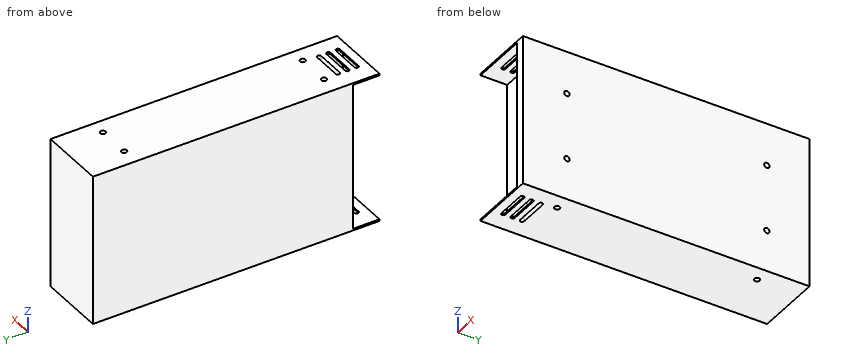
```python
from build123d import *

# Parameters (mm, degrees)
ESBO_O1_W                = 50
ESBO_O1_H                = 215
RESSALTO_EXTRUS_O1_DEPTH = 113
CORTE_EXTRUS_O1_DEPTH    = 113
ESBO_O3_W                = 110.4
ESBO_O3_H                = 20
CORTE_EXTRUS_O2_DEPTH    = 43
ESBO_O4_R                = 2
CORTE_EXTRUS_O3_DEPTH    = 113
ESBO_O5_R                = 2
CORTE_EXTRUS_O4_DEPTH    = 10
ESBO_O6_R                = 2
CORTE_EXTRUS_O5_DEPTH    = 10


with BuildPart() as part:
    # Esboço1 → Ressalto-extrusão1 (new body)
    with BuildSketch(Plane.XY):
        Rectangle(ESBO_O1_W, ESBO_O1_H)
    extrude(amount=RESSALTO_EXTRUS_O1_DEPTH)

    # Esboço2 → Corte-extrusão1 (cut)
    with BuildSketch(Plane(origin=(0, 0, 0), x_dir=(-1, 0, 0), z_dir=(0, 0, -1))):
        with BuildLine():
            Line((-11.5, -98), (10.5, -98))
            ThreePointArc((10.5, -98), (12, -99.5), (10.5, -101))
            Line((10.5, -101), (-11.5, -101))
            ThreePointArc((-11.5, -101), (-13, -99.5), (-11.5, -98))
        make_face()
        with BuildLine():
            Line((-11.5, -91), (10.5, -91))
            ThreePointArc((10.5, -91), (12, -92.5), (10.5, -94))
            Line((10.5, -94), (-11.5, -94))
            ThreePointArc((-11.5, -94), (-13, -92.5), (-11.5, -91))
        make_face()
        with BuildLine():
            Line((-11.5, -84), (10.5, -84))
            ThreePointArc((10.5, -84), (12, -85.5), (10.5, -87))
            Line((10.5, -87), (-11.5, -87))
            ThreePointArc((-11.5, -87), (-13, -85.5), (-11.5, -84))
        make_face()
    extrude(amount=-CORTE_EXTRUS_O1_DEPTH, mode=Mode.SUBTRACT)

    # Esboço3 → Corte-extrusão2 (cut)
    with BuildSketch(Plane.ZY.offset(25)):
        with Locations((56.5, -97.5)):
            Rectangle(ESBO_O3_W, ESBO_O3_H)
    extrude(amount=-CORTE_EXTRUS_O2_DEPTH, mode=Mode.SUBTRACT)

    # Esboço4 → Corte-extrusão3 (cut)
    with BuildSketch(Plane.XY.offset(113)):
        with Locations((13.5, -74.5)):
            Circle(ESBO_O4_R)
        with Locations((13.5, 75.5)):
            Circle(ESBO_O4_R)
    extrude(amount=-CORTE_EXTRUS_O3_DEPTH, mode=Mode.SUBTRACT)

    # Esboço5 → Corte-extrusão4 (cut)
    with BuildSketch(Plane.XY.offset(113)):
        with Locations((-11.5, 75.5)):
            Circle(ESBO_O5_R)
        with Locations((-11.5, -74.5)):
            Circle(ESBO_O5_R)
    extrude(amount=-CORTE_EXTRUS_O4_DEPTH, mode=Mode.SUBTRACT)

    # Esboço6 → Corte-extrusão5 (cut)
    with BuildSketch(Plane(origin=(25, 0, 0), x_dir=(0, 0, -1), z_dir=(1, 0, 0))):
        with Locations((-31, -74.5)):
            Circle(ESBO_O6_R)
        with Locations((-81, -74.5)):
            Circle(ESBO_O6_R)
        with Locations((-31, 75.5)):
            Circle(ESBO_O6_R)
        with Locations((-81, 75.5)):
            Circle(ESBO_O6_R)
    extrude(amount=-CORTE_EXTRUS_O5_DEPTH, mode=Mode.SUBTRACT)


solid = part.part
```
Source: CAD feature listing. Evaluate the final solid. Frame: model axes, mm. Coordinates: 2 decimals unless noted, no trailing zeros. Loops run counter-clockwise (first coordinate to the right, second up) from the corner with the lowest first, then second, coordinate; pieces in that order, holes last. Notation, with made-up numbers: (33.25, 49.5) - (63.25, 49.5) arc R9 cw to (63.25, 65.5) - close; hole circle Ø5 at (71, 10). An arc over 180 degrees is marked (long way). Answer as CSV lines item,"result".
1. Contact query for flat-ended pins moving along their axis: pin 1 (10 mm diameter, centred on x = -3.5, y = -99, fed in from -Z); pin 2 (24 mm diameter, centred on x = -3, z = 52.5, fed in from -Y); pin 3 (0.5 mm diameter, centred on y = 74, z = 31, fed in from +X); pin 4 (16 mm diameter, centred on y = -99, z = 38, fed in from -X). Output: stop coordinate, or through.
Established:
pin 1,"stops at z = 0"
pin 2,"stops at y = -87.5"
pin 3,"stops at x = 15"
pin 4,"stops at x = 18"
2. Section A-A (x = 1.5). Return loops of the section in (y, z).
Established:
outline,"(-107.5, 0) - (-101, 0) - (-101, 1.3) - (-107.5, 1.3) - close; (-107.5, 111.7) - (-101, 111.7) - (-101, 113) - (-107.5, 113) - close; (-98, 0) - (-94, 0) - (-94, 1.3) - (-98, 1.3) - close; (-98, 111.7) - (-94, 111.7) - (-94, 113) - (-98, 113) - close; (-91, 0) - (-87, 0) - (-87, 113) - (-91, 113) - (-91, 111.7) - (-87.5, 111.7) - (-87.5, 1.3) - (-91, 1.3) - close; (-84, 0) - (107.5, 0) - (107.5, 113) - (-84, 113) - close"
3. Section B-B (z = 75). Return loops of the section in (x, y), then the cut area to 3 significant figures.
Established:
outline,"(-25, -87.5) - (18, -87.5) - (18, -107.5) - (25, -107.5) - (25, 107.5) - (-25, 107.5) - close; hole (-10.5, -87) - (11.5, -87) arc R1.5 ccw to (11.5, -84) - (-10.5, -84) arc R1.5 ccw to start; hole circle Ø4 at (13.5, -74.5); hole circle Ø4 at (13.5, 75.5)"
area,"9,790 mm2"
4. Section C-C (x = -16.5). Return loops of the section in (y, z).
Established:
outline,"(-107.5, 0) - (107.5, 0) - (107.5, 113) - (-107.5, 113) - (-107.5, 111.7) - (-87.5, 111.7) - (-87.5, 1.3) - (-107.5, 1.3) - close"
5. Ray query, line 1 (Y direction, x = 19, z = 31); line 2 (Y direction, x = 17, z = 81); line 3 (Y direction, x = -1, z = 15.5). Return the intervals inside material, ascending.
Established:
line 1,"y = -107.5 to -76.5, -72.5 to 73.5, 77.5 to 107.5"
line 2,"y = -87.5 to -76.5, -72.5 to 73.5, 77.5 to 107.5"
line 3,"y = -87.5 to -87, -84 to 107.5"
